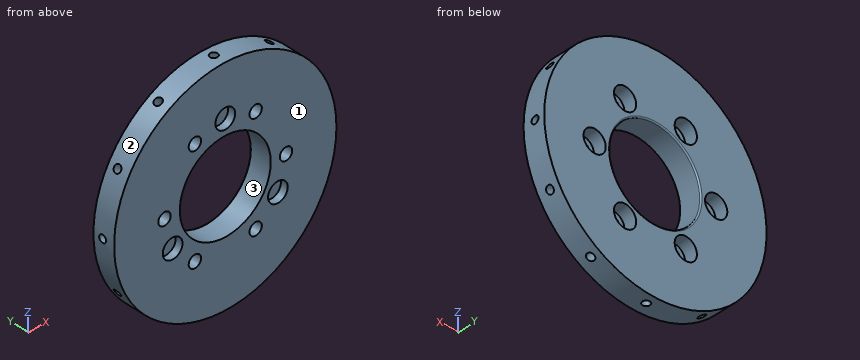
```python
from build123d import *

# Parameters (mm, degrees)
SKETCH_1_R               = 45
SKETCH_1_R_2             = 2.5
SKETCH_1_R_3             = 18.4
EXTRUDE_1_DEPTH          = 9
SKETCH_2_R               = 4
CUT_EXTRUDE_1_DEPTH      = 3
SKETCH_4_R               = 4.5
CUT_EXTRUDE_2_DEPTH      = 5.1
SKETCH_5_R               = 1.5
CUT_EXTRUDE_3_DEPTH      = 10
PATTERN_CIRCULAR_1_COUNT = 12
FILLET_1_R               = 0.5


with BuildPart() as part:
    # 草图1 → 凸台-拉伸1 (new body)
    with BuildSketch(Plane(origin=(0, 0, 0), x_dir=(1, 0, 0), z_dir=(0, 1, 0))):
        Circle(SKETCH_1_R)
        with Locations((-24.6, 0)):
            Circle(SKETCH_1_R_2, mode=Mode.SUBTRACT)
        with Locations((-12.3, 21.304224933)):
            Circle(SKETCH_1_R_2, mode=Mode.SUBTRACT)
        with Locations((12.3, 21.304224933)):
            Circle(SKETCH_1_R_2, mode=Mode.SUBTRACT)
        with Locations((24.6, 0)):
            Circle(SKETCH_1_R_2, mode=Mode.SUBTRACT)
        with Locations((12.3, -21.304224933)):
            Circle(SKETCH_1_R_2, mode=Mode.SUBTRACT)
        with Locations((-12.3, -21.304224933)):
            Circle(SKETCH_1_R_2, mode=Mode.SUBTRACT)
        Circle(SKETCH_1_R_3, mode=Mode.SUBTRACT)
    extrude(amount=EXTRUDE_1_DEPTH)

    # 草图2 → 切除-拉伸1 (cut)
    with BuildSketch(Plane.XZ):
        with Locations((-21.304224933, -12.3)):
            Circle(SKETCH_2_R)
        with Locations((0, 24.6)):
            Circle(SKETCH_2_R)
        with Locations((21.304224933, -12.3)):
            Circle(SKETCH_2_R)
    extrude(amount=-CUT_EXTRUDE_1_DEPTH, mode=Mode.SUBTRACT)

    # 草图4 → 切除-拉伸2 (cut)
    with BuildSketch(Plane(origin=(0, 9, 0), x_dir=(1, 0, 0), z_dir=(0, 1, 0))):
        with Locations((-24.6, 0)):
            Circle(SKETCH_4_R)
        with Locations((-12.3, 21.304224933)):
            Circle(SKETCH_4_R)
        with Locations((12.3, 21.304224933)):
            Circle(SKETCH_4_R)
        with Locations((24.6, 0)):
            Circle(SKETCH_4_R)
        with Locations((12.3, -21.304224933)):
            Circle(SKETCH_4_R)
        with Locations((-12.3, -21.304224933)):
            Circle(SKETCH_4_R)
    extrude(amount=-CUT_EXTRUDE_2_DEPTH, mode=Mode.SUBTRACT)

    # 草图5 → 切除-拉伸3 (cut)
    with BuildSketch(Plane(origin=(45, 0, 0), x_dir=(0, 0, -1), z_dir=(1, 0, 0))):
        with Locations((0, 5)):
            Circle(SKETCH_5_R)
    cut_extrude_3 = extrude(amount=-CUT_EXTRUDE_3_DEPTH, mode=Mode.SUBTRACT)

    # 阵列(圆周)1: 切除-拉伸3 ×12 about axis
    pattern_circular_1_axis = Axis((0, 0, 0), (0, 1, 0))
    for i in range(1, PATTERN_CIRCULAR_1_COUNT):
        add(cut_extrude_3.rotate(pattern_circular_1_axis, i * 360 / PATTERN_CIRCULAR_1_COUNT), mode=Mode.SUBTRACT)

    # 圆角1
    fillet_1_edges = [part.edges().sort_by_distance(p)[0] for p in [
        (-18.4, 9, 0),
    ]]
    fillet(fillet_1_edges, radius=FILLET_1_R)


solid = part.part
```
The model under review builds one solid part; all positions refer to its coordinate system, in mm. Face numbers are marked on the shaded views. Round coordinates to 2 decimals unless told otherwise and drop trailing zeros. Answer as a JSON object with one key per item and string values.
(1) Draft analysis for pull direction Z (two halves, no side actions). For the marked faces 1, 2 and 3, state which applies: released by +Z, released by -Z, zero draft, split by the parting line, or undercut.
Resolved:
{"face 1": "zero draft", "face 2": "split by the parting line", "face 3": "undercut"}
(2) To check wall thickness, follow line 1 along X through (y, z) = (6.2, 0); line 2 along Z through (x, y) = (12.3, 7.7); line 3 along Y through (x, z) = (0, -40.5). State the ranges of each line that lie inside material, in increasing order.
Resolved:
{"line 1": "-35 to -29.1, -20.1 to -18.4, 18.4 to 20.1, 29.1 to 35", "line 2": "-43.29 to -25.8, -16.8 to -13.68, 13.68 to 16.8, 25.8 to 43.29", "line 3": "0 to 3.5, 6.5 to 9"}
(3) Take a section at A-A on y = 1.25. Count the separate pieces of the cut face and the enclosed holes in it, and give its area (3 significant figures).
Resolved:
{"separate pieces": "1", "enclosed holes": "10", "area": "5,030 mm²"}
(4) Clearance check with flat-ended pins moving along their axes: P1, Ø1.5, axis at x = -10.5, y = 5, coming from the +Z side; P2, Ø5, axis at y = 5, z = -19.5, coming from the +X side; P3, Ø6.5, axis at x = 0, z = 25, coming from the -Y side. State where each tip first meets the part, or that it passes through.
Resolved:
{"P1": "z = 43.93", "P2": "x = 41.67", "P3": "y = 3"}
